For this review, take the finished solid that the model builds, in its own axes (mm). Face numbers are marked on the shaded views. A direction names the side the tool comes from. Coordinates: 2 decimals unless noted, no trailing zeros. Order: outer loops, then holes, each group sorted by start corner. A loop starts at its lowest first (then second) coordinate and runs counter-clockwise, first axis right, second up. Notation, with made-up numbers: (74, 61.25) -> (83, 61.25) arc R21 cw to (83, 86.25) -> close; hole circle Ø9 at (88, 68). An arc over 180 degrees is marked (long way). Answer as a JSON object with one key per item and string values. Group by question number.
1) Draft analysis for pull direction Z (two halves, no side actions). For the marked faces 1, 2 and 3, state which applies: +Z half, -Z half, draft (parallel to the pull), parting line (faces both ways), or undercut.
2) Wall thickness on L1, parallel to Y at x = 245, z = 263.9; L2, parallel to Z at x = 224.75, y = 307; L3, parallel to X at y = 288, z = 262.65: over which ranges is each line inside the solid? List them lowest first.
3) Add section A-A, the plane y = 300. Write out the cut boundary in (x, z).
4) Add section C-C, the plane z = 294.5. Write out the cut boundary in (x, y), then the cut area to 3 significant figures.
5) For pin 1 (2.5 mm diameter, centred on x = 233, y = 312, fed in from +Z); pin 2 (4.5 mm diameter, centred on y = 306.95, z = 321.4, fed in from +X); pin 3 (8 mm diameter, centred on x = 242, y = 295.5, fed in from +Z); pin 4 (1.5 mm diameter, centred on x = 226.5, z = 316.5, fed in from -Y), all flat-tipped, find the tip position at first contact; note any pin that passes through.
6) Add section B-B, the plane x = 233. Write out the cut boundary in (y, z), then the cut area to 3 significant figures.
7) Machinability: for the marked faces 4, 5, 6, 7 and 8, which of the approach directions +Z, -Z, +X, -X, +Y, -Y give a long, thin tool a straight path to every point of the face, cutting with its end or side? Answer none if there is none.
8) Add section D-D, the plane y = 288. Write out the cut boundary in (x, z).
from build123d import *

# Parameters (mm, degrees)
SKETCH1_R           = 27
BOSS_EXTRUDE1_DEPTH = 6
SKETCH2_W           = 25
SKETCH2_H           = 40
BOSS_EXTRUDE2_DEPTH = 6
SKETCH3_R           = 10
SKETCH3_R_2         = 1.45
CUT_EXTRUDE1_DEPTH  = 6.01
SKETCH4_W           = 22.01
SKETCH4_H           = 40
SKETCH4_R           = 1.7
BOSS_EXTRUDE3_DEPTH = 6


with BuildPart() as part:
    # Sketch1 → Boss-Extrude1 (new body)
    with BuildSketch(Plane(origin=(221, 0, 0), x_dir=(0, 0, -1), z_dir=(1, 0, 0))):
        with Locations((-300, 300)):
            Circle(SKETCH1_R)
    extrude(amount=BOSS_EXTRUDE1_DEPTH)

    # Sketch2 → Boss-Extrude2 (add)
    with BuildSketch(Plane(origin=(221, 0, 0), x_dir=(0, 0, -1), z_dir=(1, 0, 0))):
        with Locations((-272.5, 300)):
            Rectangle(SKETCH2_W, SKETCH2_H)
    extrude(amount=BOSS_EXTRUDE2_DEPTH)

    # Sketch3 → Cut-Extrude1 (cut)
    with BuildSketch(Plane(origin=(221, 0, 0), x_dir=(0, 0, -1), z_dir=(1, 0, 0))):
        with Locations((-300, 300)):
            Circle(SKETCH3_R)
        with Locations((-300, 322.5)):
            Circle(SKETCH3_R_2)
        with Locations((-278.601228383, 306.952882373)):
            Circle(SKETCH3_R_2)
        with Locations((-286.774831823, 281.797117627)):
            Circle(SKETCH3_R_2)
        with Locations((-313.225168177, 281.797117627)):
            Circle(SKETCH3_R_2)
        with Locations((-321.398771617, 306.952882373)):
            Circle(SKETCH3_R_2)
    extrude(amount=CUT_EXTRUDE1_DEPTH, mode=Mode.SUBTRACT)

    # Sketch4 → Boss-Extrude3 (add)
    with BuildSketch(Plane.XY.offset(260)):
        with Locations((237.995, 300)):
            Rectangle(SKETCH4_W, SKETCH4_H)
        with Locations((233, 288)):
            Circle(SKETCH4_R, mode=Mode.SUBTRACT)
        with Locations((233, 312)):
            Circle(SKETCH4_R, mode=Mode.SUBTRACT)
        with Locations((245, 288)):
            Circle(SKETCH4_R, mode=Mode.SUBTRACT)
        with Locations((245, 312)):
            Circle(SKETCH4_R, mode=Mode.SUBTRACT)
    extrude(amount=BOSS_EXTRUDE3_DEPTH)


solid = part.part
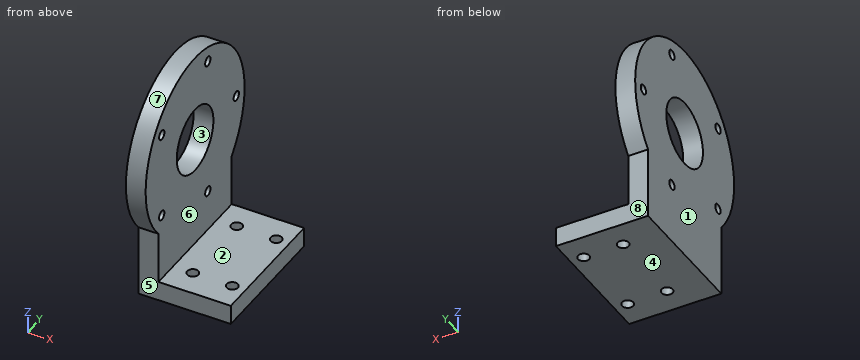
Output values:
{
 "1": {"face 1": "draft", "face 2": "+Z half", "face 3": "undercut"},
 "2": {"L1": "y = 280 to 286.3, 289.7 to 310.3, 313.7 to 320", "L2": "z = 260 to 277.15, 280.05 to 292.86, 307.14 to 319.95, 322.85 to 326.08", "L3": "x = 221 to 231.3, 234.7 to 243.3, 246.7 to 249"},
 "3": {"outline": "(221, 260) -> (249, 260) -> (249, 266) -> (227, 266) -> (227, 290) -> (221, 290) -> close; (221, 310) -> (227, 310) -> (227, 327) -> (221, 327) -> close"},
 "4": {"outline": "(221, 273.57) -> (227, 273.57) -> (227, 291.65) -> (221, 291.65) -> close; (221, 308.35) -> (227, 308.35) -> (227, 326.43) -> (221, 326.43) -> close", "area": "217 mm²"},
 "5": {"pin 1": "passes through", "pin 2": "stops at x = 227", "pin 3": "stops at z = 266", "pin 4": "stops at y = 278.07"},
 "6": {"outline": "(280, 260) -> (286.3, 260) -> (286.3, 266) -> (280, 266) -> close; (289.7, 260) -> (310.3, 260) -> (310.3, 266) -> (289.7, 266) -> close; (313.7, 260) -> (320, 260) -> (320, 266) -> (313.7, 266) -> close", "area": "199 mm²"},
 "7": {"face 4": "-Z, +X, -X, +Y, -Y", "face 5": "-Z, +X, -X, -Y", "face 6": "+Z, +X, +Y, -Y", "face 7": "+X, -X", "face 8": "-Z, +X, -X, +Y"},
 "8": {"outline": "(221, 260) -> (231.3, 260) -> (231.3, 266) -> (227, 266) -> (227, 324.19) -> (221, 324.19) -> close; (234.7, 260) -> (243.3, 260) -> (243.3, 266) -> (234.7, 266) -> close; (246.7, 260) -> (249, 260) -> (249, 266) -> (246.7, 266) -> close"}
}
